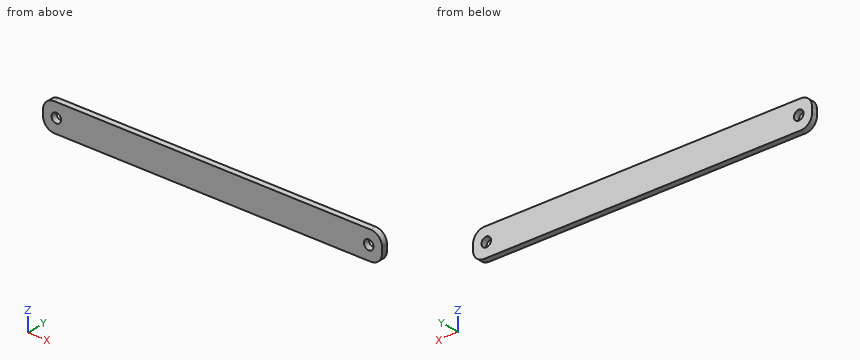
from build123d import *

# Parameters (mm, degrees)
CROQUIS1_W              = 120
CROQUIS1_H              = 10
CROQUIS1_R              = 1.7
SALIENTE_EXTRUIR1_DEPTH = 2.11
REDONDEO1_R             = 4


with BuildPart() as part:
    # Croquis1 → Saliente-Extruir1 (new body)
    with BuildSketch(Plane(origin=(0, 0, 0), x_dir=(1, 0, 0), z_dir=(0, 1, 0))):
        Rectangle(CROQUIS1_W, CROQUIS1_H)
        with Locations((-55.3, 0)):
            Circle(CROQUIS1_R, mode=Mode.SUBTRACT)
        with Locations((55.3, 0)):
            Circle(CROQUIS1_R, mode=Mode.SUBTRACT)
    extrude(amount=SALIENTE_EXTRUIR1_DEPTH)

    # Redondeo1
    redondeo1_edges = [part.edges().sort_by_distance(p)[0] for p in [
        (60, 1.055, 5),
        (-60, 1.055, 5),
        (-60, 1.055, -5),
        (60, 1.055, -5),
    ]]
    fillet(redondeo1_edges, radius=REDONDEO1_R)


solid = part.part
The model under review builds one solid part; all positions refer to its coordinate system, in mm. Coordinates: 2 decimals unless noted, no trailing zeros. Write each loop counter-clockwise with the first axis right and the second up, starting at its lowest first coordinate (ties: lowest second). Pieces come first, ordered by that corner, then holes. Notation, with made-up numbers: (-14, 41) - (-9, 41) arc R21 cw to (-9, 52) - close; hole circle Ø9 at (-31, -30.5). An arc over 180 degrees is marked (long way). Answer as a JSON object with one key per item and string values. Group by question number.
1. Clearance check with a flat-ended pin moving along its axis: pin 1 Ø4 at (x, z) = (40, 1.5) entering from -Y. State where the tip first meets the part, or that it passes through.
2. Add section B-B (y = 1.75). Give the boundary of the cut face in (x, z), plus the area to 3 significant figures.
3. To check wall thickness, follow probe 1 along X at (y, z) = (0.95, 0); probe 2 along Z at (x, y) = (-55.3, 0.75); probe 3 along X at (y, z) = (1.6, -0.5). State the ranges of each line that lie inside material, in increasing order.
4. Add section A-A (z = 0). Give the boundary of the cut face in (x, y), plus the area to 3 significant figures.
Findings:
{
 "1": {"pin 1": "y = 0"},
 "2": {"outline": "(-60, -1) arc R4 ccw to (-56, -5) - (56, -5) arc R4 ccw to (60, -1) - (60, 1) arc R4 ccw to (56, 5) - (-56, 5) arc R4 ccw to (-60, 1) - close; hole circle Ø3.4 at (-55.3, 0); hole circle Ø3.4 at (55.3, 0)", "area": "1,170 mm²"},
 "3": {"probe 1": "-60 to -57, -53.6 to 53.6, 57 to 60", "probe 2": "-5 to -1.7, 1.7 to 5", "probe 3": "-60 to -56.92, -53.68 to 53.68, 56.92 to 60"},
 "4": {"outline": "(-60, 0) - (-57, 0) - (-57, 2.11) - (-60, 2.11) - close; (-53.6, 0) - (53.6, 0) - (53.6, 2.11) - (-53.6, 2.11) - close; (57, 0) - (60, 0) - (60, 2.11) - (57, 2.11) - close", "area": "239 mm²"}
}
